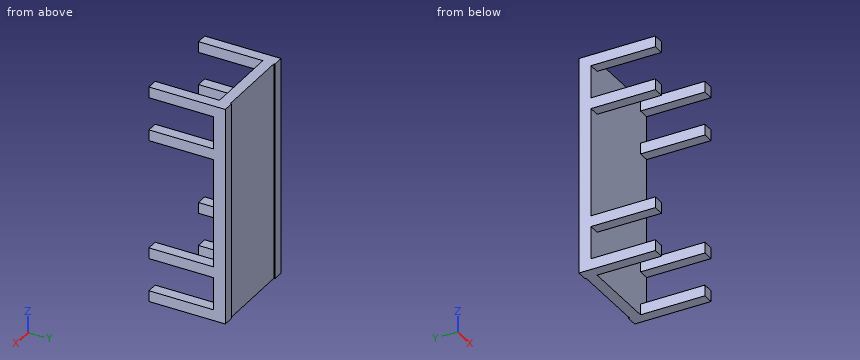
Autodesk Inventor part; units mm, degrees
ref_plane "YZ Plane" through (0, 0, 0) normal (1, 0, 0) x (0, 1, 0)
ref_plane "XZ Plane" through (0, 0, 0) normal (0, 1, 0) x (-1, 0, 0)
ref_plane "XY Plane" through (0, 0, 0) normal (0, 0, 1) x (1, 0, 0)
sketch "Sketch9" plane through (0, 0, 0) normal (0, 1, 0) x (-1, 0, 0)
  line L0 (0, 0) -> (900, 0)
  line L1 (900, 0) -> (900, -2000)
  line L2 (900, -2000) -> (0, -2000)
  line L3 (0, -2000) -> (0, 0)
  line L4 (900, -2000) -> (800, -2000)
  line L5 (800, -2000) -> (800, 3000)
  line L6 (800, 3000) -> (900, 3000)
  line L7 (900, 3000) -> (900, -2000)
  line L8 (0, -2000) -> (100, -2000)
  line L9 (100, -2000) -> (100, 0)
  line L10 (100, 0) -> (0, 0)
  line L11 (0, 0) -> (0, -2000)
  point P0 (100, -2000)
  point P1 (800, 0)
  dimension "d70" = 900
  dimension "d71" = 100
  dimension "d72" = 100
  dimension "d106" = 2000
extrude "Extrusion6" add sketch "Sketch9" along normal blind 990 contours L0 L9 L2 L3 | L0 L1 L2 L5
sketch "Sketch10" plane through (0, 0, 0) normal (1, 0, 0) x (0, 0, -1)
  line L0 (0, 0) -> (0, 990)
  line L1 (0, 990) -> (5000, 990)
  line L2 (5000, 990) -> (5000, 490)
  line L3 (5000, 490) -> (0, 490)
  line L4 (0, 490) -> (0, 990)
  line L5 (0, 990) -> (5000, 990)
  line L6 (5000, 990) -> (5000, 590)
  line L7 (5000, 590) -> (0, 590)
  line L8 (0, 590) -> (0, 990)
  line L9 (0, 990) -> (5000, 990)
  line L10 (5000, 990) -> (5000, 690)
  line L11 (5000, 690) -> (0, 690)
  line L12 (0, 690) -> (0, 990)
  line L13 (2000, 0) -> (0, 0)
  line L14 (0, 0) -> (500, 0)
  line L15 (500, 0) -> (500, 600)
  line L16 (500, 600) -> (0, 600)
  line L17 (0, 600) -> (0, 0)
  line L18 (2000, 0) -> (1500, 0)
  line L19 (1500, 0) -> (1500, 600)
  line L20 (1500, 600) -> (2000, 600)
  line L21 (2000, 600) -> (2000, 0)
  point P0 (5000, 690)
  point P1 (0, 690)
  point P2 (0, 590)
  dimension "d83" = 500
  dimension "d84" = 500
  dimension "d85" = 600
  dimension "d86" = 600
extrude "Extrusion7" add sketch "Sketch10" against normal blind 900 contours L0 L16 L15 L7 | L0 L11 L2 L7 L21 L20 L19 L15 L16 | L19 L20 L21 L7
sketch "Sketch13" plane through (0, 990, 0) normal (0, 1, 0) x (1, 0, 0)
  line L0 (-900, 2000) -> (-900, 0)
  line L1 (0, 0) -> (0, 2000)
  line L2 (-900, 0) -> (0, 0)
  line L3 (0, 0) -> (0, 2000)
  line L4 (0, 2000) -> (-900, 2000)
  line L5 (-900, 2000) -> (-900, 0)
  point P0 (0, 4500)
extrude "Extrusion9" cut sketch "Sketch13" against normal blind 290
sketch "Boceto15" plane through (0, 690, -2000) normal (0, 1, 0) x (1, 0, 0)
  line L0 (-900, 0) -> (-900, 3000)
  line L1 (0, 0) -> (-100, 0)
  line L2 (-900, 3000) -> (0, 3000)
  line L3 (0, 3000) -> (0, 0)
  line L4 (0, 0) -> (-900, 0)
  line L5 (-900, 0) -> (-900, 3000)
  point P0 (0, -2000)
  point P1 (-100, 0)
extrude "Extrusión11" cut sketch "Boceto15" against normal blind 1500
sketch "Boceto16" plane through (0, 0, 0) normal (1, 0, 0) x (0, 0, -1)
  line L0 (0, 0) -> (500, 0)
  line L1 (2000, 0) -> (0, 0)
  line L2 (2000, 0) -> (1500, 0)
  line L3 (0, 590) -> (2000, 590)
  line L4 (500, 0) -> (400, 0)
  line L5 (400, 0) -> (400, 590)
  line L6 (400, 590) -> (500, 590)
  line L7 (500, 590) -> (500, 0)
  line L8 (0, 0) -> (100, 0)
  line L9 (100, 0) -> (100, 590)
  line L10 (100, 590) -> (0, 590)
  line L11 (0, 590) -> (0, 0)
  line L12 (2000, 0) -> (1900, 0)
  line L13 (1900, 0) -> (1900, 590)
  line L14 (1900, 590) -> (2000, 590)
  line L15 (2000, 590) -> (2000, 0)
  line L16 (1500, 0) -> (1600, 0)
  line L17 (1600, 0) -> (1600, 590)
  line L18 (1600, 590) -> (1500, 590)
  line L19 (1500, 590) -> (1500, 0)
  point P0 (1600, 590)
  point P1 (100, 590)
  point P2 (1500, 590)
  dimension "d110" = 500
  dimension "d111" = 500
  dimension "d112" = 100
  dimension "d113" = 100
  dimension "d114" = 100
  dimension "d115" = 100
extrude "Extrusión12" cut sketch "Boceto16" against normal blind 1500 contours L9 L3 L5 L0 | L7 L3 L19 L1 | L17 L3 L13 L1
properties part number "B_Transportadora_Recta_5m" material "Aluminum 6061"
Geometry check sheet. Reference: the model listing, model coordinates, mm. Coordinates: 2 decimals unless noted, no trailing zeros. Order: outer loops, then holes, each group sorted by start corner. A loop starts at its lowest first (then second) coordinate and runs counter-clockwise, first axis right, second up. Notation, with made-up numbers: M 16,-21.75 L 67,-21.75 A18 cw 67,-11.75 Z; hole C 72,84.25 d3. An arc over 180 degrees is marked long. Answer as a JSON object with one key per item and string values.
Q1. Cross-section at D-D on z = -481.5. Record the cut outline in (x, y).
Results are:
{"outline": "M -900,0 L -800,0 L -800,590 L -100,590 L -100,0 L 0,0 L 0,700 L -100,700 L -100,690 L -800,690 L -800,700 L -900,700 Z"}
Q2. Cross-section at A-A on y = 153.5. Give the number of separate pieces and of enclosed holes in the cut face, and give its area (3 significant figures).
Results are:
{"separate pieces": "8", "enclosed holes": "0", "area": "80,000 mm²"}
Q3. Depth check by flat-ended pin: pin 1 Ø1 at (y, z) = (299.5, -487) entering from +X; pin 2 Ø8 at (x, z) = (-120, -1490.5) entering from +Y. Enter the tip coordinate at first touch or a pass-through.
Results are:
{"pin 1": "stops at x = 0", "pin 2": "stops at y = 690"}
Q4. Cross-section at C-C on x = -65.5. Record the cut outline in (y, z).
Results are:
{"outline": "M 0,-2000 L 700,-2000 L 700,0 L 0,0 L 0,-100 L 590,-100 L 590,-400 L 0,-400 L 0,-500 L 590,-500 L 590,-1500 L 0,-1500 L 0,-1600 L 590,-1600 L 590,-1900 L 0,-1900 Z"}
Q5. Scan lines: line 1 (Z direction, x = -811.5, y = 43); line 2 (X direction, y = 172, z = -1527.5); line 3 (Y direction, x = -133, z = -1222). Record each from-to range of solid material in increasing order.
Results are:
{"line 1": "z = -2000 to -1900, -1600 to -1500, -500 to -400, -100 to 0", "line 2": "x = -900 to -800, -100 to 0", "line 3": "y = 590 to 690"}
Q6. Cross-section at B-B on z = -276.5. Record the cut outline in (x, y), and give its area (3 significant figures).
Results are:
{"outline": "M -900,590 L 0,590 L 0,700 L -100,700 L -100,690 L -800,690 L -800,700 L -900,700 Z", "area": "92,000 mm²"}
